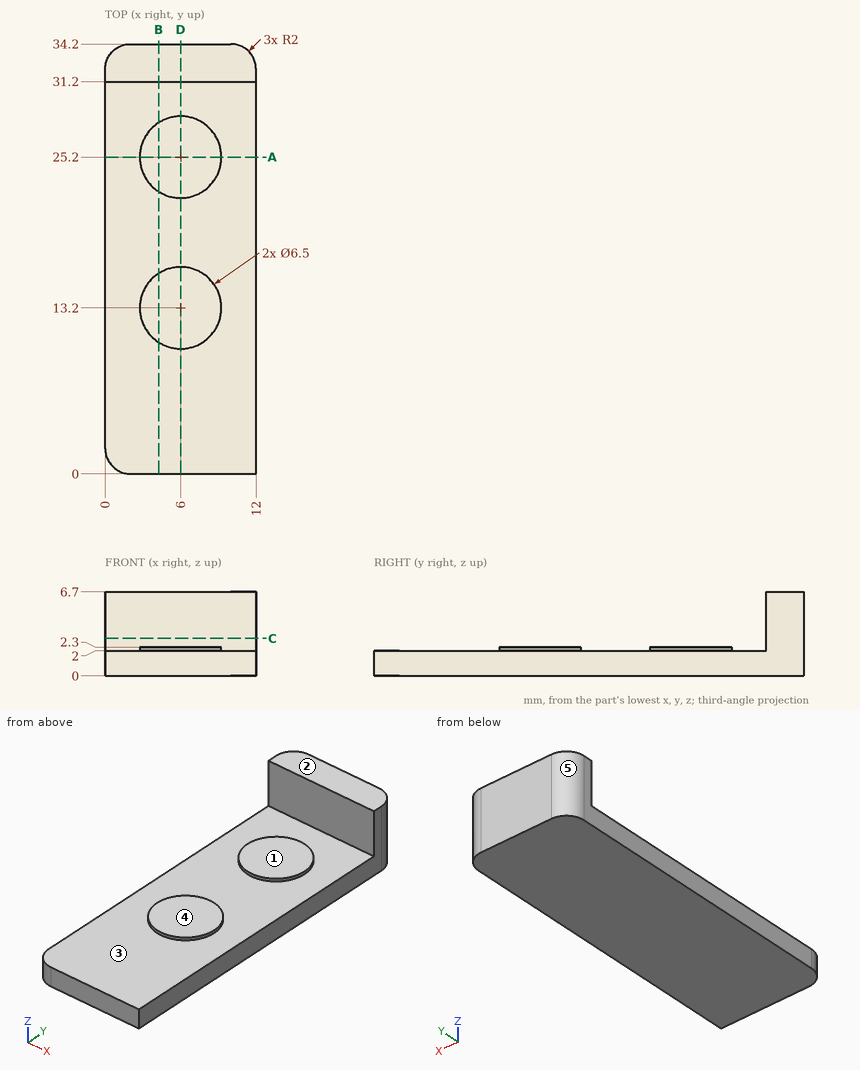
Can you work these out from the drawing? Everything is in mm from the part's minimum corner. A direction names the side the tool comes from. Coordinates: 2 decimals unless noted, no trailing zeros. Write each loop counter-clockwise with the first axis right and the second up, starting at its lowest first coordinate (ties: lowest second). Pieces come first, ordered by that corner, then holes. Notation, with made-up numbers: (-19, 68) -> (36, 68) arc R21 ccw to (36, 99) -> close; hole circle Ø11 at (57.5, 32). An arc over 180 degrees is marked (long way). Write each question's results on one line, items separated by ' | '. Start each with the question number.
Item 1: I'm going to push flat-ended pins straight in: P1, Ø4, axis at x = 2.5, y = 10, coming from the +Z side; P2, Ø2.5, axis at x = 8, z = 4, coming from the -Y side. Where does each tip first touch, or does it pass through?
Item 2: Thinking about a two-plate mould opening in Y: for the marked faces 3, 4 and 5, which applies, released by +Y, released by -Y, zero draft, split by the parting line, or undercut?
Item 3: If we section it at A-A, the plane y = 25.2: Write out the boundary of the cut face in (x, z), and give its area (4 significant figures).
Item 4: Please list where these lines run through material, in increasing order: probe 1 along Y at (x, z) = (7, 4.25); probe 2 along Z at (x, y) = (8.5, 4); probe 3 along Z at (x, y) = (3.5, 23.5).
Item 5: If we section it at B-B, the plane x = 4.25: Write out the boundary of the cut face in (y, z), and give its area (3 significant figures).
Item 6: On a 3-axis mill with a long thin cutter (end or side, diameter ignored), from which of +Z, -Z, +X, -X, +Y, -Y can I reach the whole of each face in a straight line? I mean the marked faces 1 and 2. Say none if no direction works.
Item 7: If we section it at C-C, the plane z = 3: Write out the boundary of the cut face in (x, y), and give its area (3 significant figures).
Item 8: If we section it at D-D, the plane x = 6: Write out the boundary of the cut face in (y, z).
Answer block:
1) P1: z = 2.3 | P2: y = 31.2
2) face 3: undercut | face 4: zero draft | face 5: released by +Y
3) outline: (0, 0) -> (12, 0) -> (12, 2) -> (9.25, 2) -> (9.25, 2.3) -> (2.75, 2.3) -> (2.75, 2) -> (0, 2) -> close | area: 25.95 mm²
4) probe 1: 31.2 to 34.2 | probe 2: 0 to 2 | probe 3: 0 to 2.3
5) outline: (0, 0) -> (34.2, 0) -> (34.2, 6.7) -> (31.2, 6.7) -> (31.2, 2) -> (27.94, 2) -> (27.94, 2.3) -> (22.46, 2.3) -> (22.46, 2) -> (15.94, 2) -> (15.94, 2.3) -> (10.46, 2.3) -> (10.46, 2) -> (0, 2) -> close | area: 85.8 mm²
6) face 1: +Z, +X, -X, -Y | face 2: +Z, +X, -X, +Y, -Y
7) outline: (0, 31.2) -> (12, 31.2) -> (12, 32.2) arc R2 ccw to (10, 34.2) -> (2, 34.2) arc R2 ccw to (0, 32.2) -> close | area: 34.3 mm²
8) outline: (0, 0) -> (34.2, 0) -> (34.2, 6.7) -> (31.2, 6.7) -> (31.2, 2) -> (28.45, 2) -> (28.45, 2.3) -> (21.95, 2.3) -> (21.95, 2) -> (16.45, 2) -> (16.45, 2.3) -> (9.95, 2.3) -> (9.95, 2) -> (0, 2) -> close
